For this review, take the finished solid that the model builds, in its own axes (mm). A direction names the side the tool comes from. Give positions to 0.01 mm unless a question says otherwise; leave off trailing zeros. Write each loop counter-clockwise with the first axis right and the second up, starting at its lowest first coordinate (ties: lowest second). Pieces come first, ordered by that corner, then holes. Notation, with made-up numbers: M 21,0 L 32,0 A10 cw 32,16 Z; hole C -7,16 d9. An arc over 180 degrees is marked long. Write item = value, one per line.
Autodesk Inventor part; units mm, degrees
ref_plane "YZ Plane" through (0, 0, 0) normal (1, 0, 0) x (0, 1, 0)
ref_plane "XZ Plane" through (0, 0, 0) normal (0, 1, 0) x (-1, 0, 0)
ref_plane "XY Plane" through (0, 0, 0) normal (0, 0, 1) x (1, 0, 0)
sketch "Sketch1" plane through (0, 0, 0) normal (0, 1, 0) x (-1, 0, 0)
  line L0 (0, 0) -> (37, 0)
  line L1 (37, 0) -> (37, -12)
  line L2 (37, -12) -> (0, -12)
  line L3 (0, -12) -> (0, 0)
  dimension "d0" = 12
  dimension "d1" = 37
extrude "Extrusion1" add sketch "Sketch1" along normal blind 34
fillet "Fillet1" radius 2 8 edges at (0, 17, 0) (0, 17, -12) (-37, 17, 0) (-37, 17, -12) (-18.5, 0, 0) (-18.5, 0, -12) (0, 0, -6) (-37, 0, -6)
shell "Shell1" thickness 0.2 removed faces 1 at (-24, 34, -4)
sketch "Sketch2" plane through (0, 2, -10) normal (1, 0, 0) x (0, 0, -1)
  line L0 (0, 32) -> (-8, 32)
  line L1 (0, 32) -> (0, 0)
  line L2 (-8, 32) -> (0, 32)
  line L3 (0, 32) -> (0, 31)
  line L4 (0, 31) -> (-8, 31)
  line L5 (-8, 31) -> (-8, 32)
  point P0 (-10, -2)
  dimension "d6" = 1
extrude "Extrusion2" cut sketch "Sketch2" against normal blind 10
properties part number "Down_Case"
1. We need section B-B, the plane z = -2.75. Write out the cut boundary in (x, y), then the cut area to 3 significant figures.
Responses:
outline = M -37,2 A2 ccw -35,0 L -2,0 A2 ccw 0,2 L 0,33 L -0.2,33 L -0.2,2 A1.8 cw -2,0.2 L -35,0.2 A1.8 cw -36.8,2 L -36.8,34 L -37,34 Z
area = 20.4 mm2
2. We need section A-A, the plane y = 28. Write out the cut boundary in (x, z).
Responses:
outline = M -37,-10 A2 ccw -35,-12 L -2,-12 A2 ccw 0,-10 L 0,-2 A2 ccw -2,0 L -35,0 A2 ccw -37,-2 Z; hole M -36.8,-10 A1.8 ccw -35,-11.8 L -2,-11.8 A1.8 ccw -0.2,-10 L -0.2,-2 A1.8 ccw -2,-0.2 L -35,-0.2 A1.8 ccw -36.8,-2 Z
3. The part is to be moulded in two halves that separate along X. For faces 1 (the face through (-0.2, 17, -6)), 2 (the face through (-18, 0, -6)), 3 (the face through (-36.4, 18.22, -11.43)), say which applies: +X half, -X half, draft (parallel to the pull), parting line (faces both ways), or undercut.
Responses:
face_1 = undercut
face_2 = draft
face_3 = -X half
4. We need section C-C, the plane x = -27. Write out the cut boundary in (y, z), then the cut area to 3 significant figures.
Responses:
outline = M 0,-10 A2 ccw 2,-12 L 34,-12 L 34,-11.8 L 2,-11.8 A1.8 cw 0.2,-10 L 0.2,-2 A1.8 cw 2,-0.2 L 34,-0.2 L 34,0 L 2,0 A2 ccw 0,-2 Z
area = 15.6 mm2
5. For line 1 along Z through (x, y) = (-7.5, 15.5); line 2 along X through (y, z) = (7.5, -4.5); line 3 along Y through (x, z) = (-7, -5.5), list the stretches that pass through material, from the lowest coordinate up. Write a range as from..to.
Responses:
line_1 = -12..-11.8, -0.2..0
line_2 = -37..-36.8, -0.2..0
line_3 = 0..0.2
6. Machinability: for faces 4 (the face through (-36.8, 18, -6)), 5 (the face through (-0.6, 18.22, -0.57)), which of the approach directions +Z, -Z, +X, -X, +Y, -Y give a long, thin tool a straight path to every point of the face, cutting with its end or side? Answer none if there is none.
Responses:
face_4 = +Y
face_5 = +Z, +X, +Y, -Y
